Build history of the part. All positions in model axes, mm. Give positions to 0.01 mm unless a question says otherwise; leave off trailing zeros. Write each loop counter-clockwise with the first axis right and the second up, starting at its lowest first coordinate (ties: lowest second). Pieces come first, ordered by that corner, then holes. Notation, with made-up numbers: (-8.75, 77) -> (15.25, 77) arc R8 ccw to (15.25, 81) -> close; hole circle Ø2 at (-26.75, 18). An arc over 180 degrees is marked (long way). One line per question, with ' | ' between items. Start each with the question number.
(1) Band-saw the part on C-C, the plane y = 1.55. Give the cut face in (x, z), and give its area (3 significant figures).
(2) Pin check, flat tip, straight feed: P1, Ø2, axis at y = 2, z = 1.5, coming from the -X side. Stop position of the tip, or through.
(3) Drill centre lines: probe 1 along X at (y, z) = (-0.1, 0.4); probe 2 along Y at (x, z) = (0, 1.7); probe 3 along X at (y, z) = (-1.7, 2.75). Where is each one in solid material? Low to high. Write a range as from..to.
(4) Band-saw the part on A-A, the plane y = 0. Give the cut face in (x, z).
(5) Pull direction X, two halves, no side cores. Call faces 1 (the cylindrical face through (-39, 0, 2)), 2 (the flat face through (-18, 3, 2)), 3 (the cylindrical face through (0, -2, 2)): released by +X, released by -X, zero draft, split by the parting line, or undercut.
(6) Band-saw the part on B-B, the plane z = 1.4. Give the cut face in (x, y), and give its area (3 significant figures).
from build123d import *

# Parameters (mm, degrees)
SKETCH1_R           = 2
BOSS_EXTRUDE1_DEPTH = 4


with BuildPart() as part:
    # Sketch1 → Boss-Extrude1 (new body)
    with BuildSketch(Plane.XY):
        with BuildLine():
            Line((-36, 3), (0, 3))
            ThreePointArc((0, 3), (3, 0), (0, -3))
            Line((0, -3), (-36, -3))
            ThreePointArc((-36, -3), (-39, 0), (-36, 3))
        make_face()
        Circle(SKETCH1_R, mode=Mode.SUBTRACT)
        with Locations(Location((-36, 0, 0), (0, 0, 180))):
            Circle(SKETCH1_R, mode=Mode.SUBTRACT)
    extrude(amount=BOSS_EXTRUDE1_DEPTH)


solid = part.part
Results:
1) outline: (-38.57, 0) -> (-37.26, 0) -> (-37.26, 4) -> (-38.57, 4) -> close; (-34.74, 0) -> (-1.26, 0) -> (-1.26, 4) -> (-34.74, 4) -> close; (1.26, 0) -> (2.57, 0) -> (2.57, 4) -> (1.26, 4) -> close | area: 144 mm²
2) P1: stops at x = -38.83
3) probe 1: x = -39..-38, -34..-2, 2..3 | probe 2: y = -3..-2, 2..3 | probe 3: x = -38.47..-37.05, -34.95..-1.05, 1.05..2.47
4) outline: (-39, 0) -> (-38, 0) -> (-38, 4) -> (-39, 4) -> close; (-34, 0) -> (-2, 0) -> (-2, 4) -> (-34, 4) -> close; (2, 0) -> (3, 0) -> (3, 4) -> (2, 4) -> close
5) face 1: released by -X | face 2: zero draft | face 3: undercut
6) outline: (-36, -3) -> (0, -3) arc R3 ccw to (0, 3) -> (-36, 3) arc R3 ccw to start; hole circle Ø4 at (-36, 0); hole circle Ø4 at (0, 0) | area: 219 mm²
